from build123d import *

# Parameters (mm, degrees)
F0_W           = 100
F0_H           = 25
F1_DEPTH       = 50
F2_SIZE        = 2
F3_R           = 12.5
F4_DEPTH       = 27.5
F5_R           = 5
F7_D           = 3.2
F7_CSINK_D     = 8.96
F7_CSINK_ANGLE = 90


with BuildPart() as f1:
    # F0 (on Front) → F1 (new body)
    with BuildSketch(Plane.XZ):
        with Locations((0.2977304684, -1.6892874761)):
            Rectangle(F0_W, F0_H)
    extrude(amount=F1_DEPTH)

    # F2
    f2_edges = [f1.edges().sort_by_distance(p)[0] for p in [
        (0.29773, -50, 10.810713),
    ]]
    chamfer(f2_edges, length=F2_SIZE)

    # F3 (on face) → F4 (join)
    with BuildSketch(Plane.XY.offset(10.8107125239)):
        with Locations((0.2977304684, -25)):
            Circle(F3_R)
    extrude(amount=F4_DEPTH)

    # F5
    f5_edges = [f1.edges().sort_by_distance(p)[0] for p in [
        (-12.20227, -25, 38.310713),
    ]]
    fillet(f5_edges, radius=F5_R)

    # F7 (through all)
    with Locations(Plane.XY.offset(38.3107125239)):
        with Locations((0.2977304684, -25)):
            CounterSinkHole(F7_D / 2, F7_CSINK_D / 2, counter_sink_angle=F7_CSINK_ANGLE)


solid = f1.part
The listing builds one solid part. Answer for the finished solid, in the listing's coordinates (mm). A direction names the side the tool comes from. Round coordinates to 2 decimals unless told otherwise and drop trailing zeros. Write each loop counter-clockwise with the first axis right and the second up, starting at its lowest first coordinate (ties: lowest second). Pieces come first, ordered by that corner, then holes. Notation, with made-up numbers: (79, 87.5) - (138, 87.5) arc R17 cw to (138, 99.5) - close; hole circle Ø7 at (18.25, 7). An arc over 180 degrees is marked (long way). Use a Markdown table: item, result. Add a question column.
1. Consider line 1 (X direction, y = -25, z = 5); line 2 (X direction, y = -26, z = 15.5); line 3 (Z direction, x = -10, y = -12). Determine where each line is inside the solid, lowest interval first.
2. Flat-ended cylindrical pins translate along their axes: P1, Ø2.5, axis at x = 0.3, y = -25, coming from the +Z side; P2, Ø5, axis at x = 1, z = 18.5, coming from the -Y side; P3, Ø1, axis at x = 16, y = -23, coming from the +Z side; P4, Ø12, axis at x = 22, z = 5.5, coming from the +Y side. Find the tip coordinate at first contact, or state that the pin passes through.
3. The part is cut by section C-C (z = 30). Write down the section's boundary in (x, y), and give its area (3 significant figures).
4. A tool of negligible diameter and unlimited length cuts with its end or side. For faces 4 (the face through (-2.412, -37.203, 21.903)), 5 (the face through (0, -19, -14.189)), from which of +Z, -Z, +X, -X, +Y, -Y can it reach the whole face along a straight path? Write none if from no direction.
5. For a pull along X with two mould halves and no side action, classify faces 1 (the face through (-49.702, -25, -2)), 2 (the face through (4, -28, 38.311)), 3 (the face through (-0.51, -26.54, 35.57)) as +X half, -X half, draft (parallel to the pull), parting line (faces both ways), or undercut.
6. The part is cut by section B-B (x = 18). Write down the section's boundary in (y, z).
7. The part is cut by section A-A (y = -25). Write down the section's boundary in (x, z).
8. The part is cut by section D-D (y = -9.5). Write down the section's boundary in (x, z).
Reported:
| question | item | result |
|---|---|---|
| 1 | line 1 | -49.7 to -1.3, 1.9 to 50.3 |
| 1 | line 2 | -12.16 to -0.95, 1.55 to 12.76 |
| 1 | line 3 | -14.19 to 10.81 |
| 2 | P1 | through |
| 2 | P2 | y = -37.5 |
| 2 | P3 | z = 10.81 |
| 2 | P4 | y = 0 |
| 3 | outline | circle Ø25 at (0.3, -25); hole circle Ø3.2 at (0.3, -25) |
| 3 | area | 483 mm^2 |
| 4 | face 4 | +Z |
| 4 | face 5 | -Z, +X, -X, +Y, -Y |
| 5 | face 1 | -X half |
| 5 | face 2 | draft |
| 5 | face 3 | undercut |
| 6 | outline | (-50, -14.19) - (0, -14.19) - (0, 10.81) - (-48, 10.81) - (-50, 8.81) - close |
| 7 | outline | (-49.7, -14.19) - (-1.3, -14.19) - (-1.3, 35.43) - (-4.18, 38.31) - (-7.2, 38.31) arc R5 ccw to (-12.2, 33.31) - (-12.2, 10.81) - (-49.7, 10.81) - close; (1.9, -14.19) - (50.3, -14.19) - (50.3, 10.81) - (12.8, 10.81) - (12.8, 33.31) arc R5 ccw to (7.8, 38.31) - (4.78, 38.31) - (1.9, 35.43) - close |
| 8 | outline | (-49.7, -14.19) - (50.3, -14.19) - (50.3, 10.81) - (-49.7, 10.81) - close |
